from build123d import *

# Parameters (mm, degrees)
ESBO_O1_W                        = 72.2
ESBO_O1_H                        = 43
RESSALTO_EXTRUS_O1_DEPTH         = 8
ESBO_O2_R                        = 11
ESBO_O2_R_2                      = 1.5
CORTE_EXTRUS_O1_DEPTH            = 9
REBAIXO_PARA_SHCS_M21_AT_2_COUNT = 2
REBAIXO_PARA_SHCS_M21_AT_2_PITCH = 20


with BuildPart() as part:
    # Esboço1 → Ressalto-extrusão1 (new body)
    with BuildSketch(Plane.XY):
        Rectangle(ESBO_O1_W, ESBO_O1_H)
    extrude(amount=RESSALTO_EXTRUS_O1_DEPTH)

    # Esboço2 → Corte-extrusão1 (cut, through all)
    with BuildSketch(Plane.XY.offset(8)):
        with Locations((-21.1, 7)):
            Circle(ESBO_O2_R)
        with Locations((15, -2.6)):
            Circle(ESBO_O2_R)
        with Locations((-0.5, 12.9)):
            Circle(ESBO_O2_R_2)
        with Locations((30.5, 12.9)):
            Circle(ESBO_O2_R_2)
        with Locations((30.5, -18.1)):
            Circle(ESBO_O2_R_2)
        with Locations((-0.5, -18.1)):
            Circle(ESBO_O2_R_2)
    extrude(amount=-CORTE_EXTRUS_O1_DEPTH, mode=Mode.SUBTRACT)

    # Esboço6 → Rebaixo para SHCS M21 (revolve, cut)
    with BuildSketch(Plane(origin=(-31.1, -19, 8), x_dir=(0, -1, 0), z_dir=(1, 0, 0))):
        Polygon((0, 0), (0, 8), (1.2, 8), (1.2, 2), (2.2, 2), (2.2, 0.025), (2.225, 0), align=None)
    rebaixo_para_shcs_m21 = revolve(axis=Axis((-31.1, -19, 14.35), (0, 0, -1)), mode=Mode.SUBTRACT)

    # Rebaixo para SHCS M21 at 2: Rebaixo para SHCS M21 ×2
    with Locations(*[(i * REBAIXO_PARA_SHCS_M21_AT_2_PITCH, 0, 0) for i in range(1, REBAIXO_PARA_SHCS_M21_AT_2_COUNT)]):
        add(rebaixo_para_shcs_m21, mode=Mode.SUBTRACT)


solid = part.part
Model file for the job. Use its own axes, mm. A direction names the side the tool comes from. Give positions to 0.01 mm unless a question says otherwise; leave off trailing zeros. Order: outer loops, then holes, each group sorted by start corner. A loop starts at its lowest first (then second) coordinate and runs counter-clockwise, first axis right, second up. Notation, with made-up numbers: M 25.5,12 L 66.5,12 A30 ccw 66.5,48 Z; hole C 8.25,15.25 d3. An arc over 180 degrees is marked long. Put each result on its own line as item: value. Start each with the question number.
(1) Drill centre lines: L1, parallel to Y at x = -0.5, z = 4; L2, parallel to X at y = 2.5, z = 4; L3, parallel to X at y = 14, z = 2.25. Where is each one in solid material? Low to high. Write a range as [from, to].
(2) Band-saw the part on B-B on z = 1.75. Count the separate pieces of the cut face and the enclosed holes in it, then the cut area to 3 significant figures.
(3) Band-saw the part on A-A on x = -21.1. Give the cut face in (y, z).
(4) Pull direction X, two halves, no side cores. Call faces 3 (the face through (36.1, 0, 4)), 4 (the face through (-10.035, -19.554, 3.042)), 5 (the face through (-1, 21.5, 4)), 6 (the face through (29, 12.97, 4.06)): released by +X, released by -X, zero draft, split by the parting line, or undercut.
(5) Tool access for faces 1 (the face through (-10, -18, 6)), 2 (the face through (-23.48, -3.74, 4.06)): list every direction of +Z, -Z, +X, -X, +Y, -Y with a clear straight run to the whole face (end or side of a thin tool).
(6) Band-saw the part on C-C on x = -11.1. Give the cut face in (y, z) (3 decimals).
(7) Pin check, flat tips, straight feed: pin 1 Ø1.3 at (x, y) = (-31, -18.5) entering from +Z; pin 2 Ø5 at (x, y) = (-10.5, -19) entering from +Z; pin 3 Ø4 at (x, y) = (-11.1, -19) entering from +Z. Stop position of each tip, or through.
(8) Band-saw the part on D-D on y = -5. Give the cut face in (x, z), then the cut area to 3 significant figures.
Results below:
1. L1: y = [-21.5, -19.6], [-16.6, 11.4], [14.4, 21.5]
1. L2: x = [-36.1, -31.14], [-11.06, 5.25], [24.75, 36.1]
1. L3: x = [-36.1, -29.59], [-12.61, -1.52], [0.52, 29.48], [31.52, 36.1]
2. separate pieces: 1
2. enclosed holes: 8
2. area: 2,310 mm2
3. outline: M -21.5,0 L -4,0 L -4,8 L -21.5,8 Z; M 18,0 L 21.5,0 L 21.5,8 L 18,8 Z
4. face 3: released by +X
4. face 4: undercut
4. face 5: zero draft
4. face 6: undercut
5. face 1: +Z
5. face 2: +Z, -Z
6. outline: M -21.5,0 L -20.2,0 L -20.2,6 L -21.2,6 L -21.2,7.975 L -21.225,8 L -21.5,8 Z; M -17.8,0 L 2.417,0 L 2.417,8 L -16.775,8 L -16.8,7.975 L -16.8,6 L -17.8,6 Z; M 11.583,0 L 21.5,0 L 21.5,8 L 11.583,8 Z
7. pin 1: passes through
7. pin 2: stops at z = 8
7. pin 3: stops at z = 6
8. outline: M -36.1,0 L 4.27,0 L 4.27,8 L -36.1,8 Z; M 25.73,0 L 36.1,0 L 36.1,8 L 25.73,8 Z
8. area: 406 mm2
